Could you check a few things on this model? Use its own coordinates, in mm. A direction names the side the tool comes from. Give positions to 0.01 mm unless a question says otherwise; leave off trailing zeros. Loops run counter-clockwise (first coordinate to the right, second up) from the corner with the lowest first, then second, coordinate; pieces in that order, holes last. Notation, with made-up numbers: (2.5, 84.25) - (54.5, 84.25) arc R35 cw to (54.5, 121.25) - close; hole circle Ø4 at (48, 12). An arc over 180 degrees is marked (long way). Use CSV: the item, a comma, the result in double quotes.
from build123d import *

# Parameters (mm, degrees)
SKETCH1_W                         = 25.4
SKETCH1_H                         = 50.8
SKETCH1_W_2                       = 19.05
SKETCH1_H_2                       = 44.45
EXTRUDE_THIN1_DEPTH               = 501.65
F_3_16_0_1875_DIAMETER_HOLE1_D    = 4.7625
F_3_16_0_195_DIAMETER_HOLE1_D     = 4.953
F_3_16_0_195_DIAMETER_HOLE1_DEPTH = 3.175
F_1_4_0_25_DIAMETER_HOLE1_D       = 6.35
F_1_4_0_25_DIAMETER_HOLE1_DEPTH   = 25.4
F_1_4_0_25_DIAMETER_HOLE1_TIP     = 1.907732465
F_1_4_CLEARANCE_HOLE1_D           = 6.7564
F_1_4_CLEARANCE_HOLE1_DEPTH       = 38.1
F_1_4_CLEARANCE_HOLE1_TIP         = 2.029827343


with BuildPart() as part:
    # Sketch1 → Extrude-Thin1 (new body)
    with BuildSketch(Plane.XY):
        Rectangle(SKETCH1_W, SKETCH1_H)
        Rectangle(SKETCH1_W_2, SKETCH1_H_2, mode=Mode.SUBTRACT)
    extrude(amount=EXTRUDE_THIN1_DEPTH)

    # 3/16 (0.1875) Diameter Hole1 (through all)
    with Locations(Plane(origin=(0, 25.4, 495.3), x_dir=(0, 0, 1), z_dir=(0, 1, 0))):
        with Locations((0, 0), (-488.95, 0), (-463.55, 0), (-438.15, 0), (-25.4, 0), (-50.8, 0)):
            Hole(F_3_16_0_1875_DIAMETER_HOLE1_D / 2)

    # 3/16 (0.195) Diameter Hole1
    with Locations(Plane(origin=(0, -25.4, 0), x_dir=(-1, 0, 0), z_dir=(0, -1, 0))):
        with Locations((-3.175, -85.719336228), (3.175, -111.119336228), (-3.175, -136.519336228), (3.175, -161.919336228), (-3.175, -187.319336228), (3.175, -212.719336228), (-3.175, -238.119336228), (3.175, -263.519336228), (-3.175, -288.919336228), (3.175, -314.319336228), (-3.175, -339.719336228), (3.175, -365.119336228), (3.175, -415.919336228), (-3.175, -390.519336228)):
            Hole(F_3_16_0_195_DIAMETER_HOLE1_D / 2, depth=F_3_16_0_195_DIAMETER_HOLE1_DEPTH)

    # 1/4 (0.25) Diameter Hole1
    with Locations(Plane(origin=(0, 25.4, 0), x_dir=(1, 0, 0), z_dir=(0, 1, 0))):
        with Locations((0, -200.464463093), (0, -422.731), (0, -327.481), (0, -86.154539829)):
            Hole(F_1_4_0_25_DIAMETER_HOLE1_D / 2, depth=F_1_4_0_25_DIAMETER_HOLE1_DEPTH)
            with Locations((0, 0, -(F_1_4_0_25_DIAMETER_HOLE1_DEPTH + F_1_4_0_25_DIAMETER_HOLE1_TIP / 2))):  # 118° drill point
                Cone(0, F_1_4_0_25_DIAMETER_HOLE1_D / 2, F_1_4_0_25_DIAMETER_HOLE1_TIP, mode=Mode.SUBTRACT)

    # 1/4 Clearance Hole1
    with Locations(Plane(origin=(-381, 25.4, 250.825), x_dir=(1, 0, 0), z_dir=(0, 1, 0))):
        with Locations((381, 82.55), (381, 98.425), (381, 114.3), (381, -146.05), (381, -130.175), (381, -114.3), (-381, -146.05), (-381, -130.175), (-381, -114.3), (-381, 82.55), (-381, 98.425), (-381, 114.3)):
            Hole(F_1_4_CLEARANCE_HOLE1_D / 2, depth=F_1_4_CLEARANCE_HOLE1_DEPTH)
            with Locations((0, 0, -(F_1_4_CLEARANCE_HOLE1_DEPTH + F_1_4_CLEARANCE_HOLE1_TIP / 2))):  # 118° drill point
                Cone(0, F_1_4_CLEARANCE_HOLE1_D / 2, F_1_4_CLEARANCE_HOLE1_TIP, mode=Mode.SUBTRACT)


solid = part.part
1) Which directions (+Z, -Z, +X, -X, +Y, -Y) give clear straight access to the entire face, cutting with the end or side of a thin tool? Please do faces 1 (the flat face through (0, -22.225, 247)), 2 (the flat face through (12.7, 0, 247)).
Answer below:
face 1,"+Z, -Z"
face 2,"+Z, -Z, +X, +Y, -Y"
2) Suppose I cut it at A-A (y = -17). Please give me the cut outline in (x, z) (3 decimals), plus the area to 3 significant figures.
Answer below:
outline,"(-12.7, 0) - (-9.525, 0) - (-9.525, 501.65) - (-12.7, 501.65) - close; (9.525, 0) - (12.7, 0) - (12.7, 501.65) - (9.525, 501.65) - close"
area,"3,190 mm2"
3) We'd pull the mould along X, two halves only. Please class faces 3 (the flat face through (0, 25.4, 247)), 4 (the flat face through (-9.525, 0, 247)), 5 (the flat face through (-12.7, 0, 247)): +X half, -X half, draft (parallel to the pull), parting line (faces both ways), or undercut.
Answer below:
face 3,"draft"
face 4,"undercut"
face 5,"-X half"
4) I need wall thicknesses on line 1 along Y through (x, z) = (0.25, 457.5) (3 decimals); line 2 along X through (y, z) = (-9, 42) (3 decimals); line 3 along X through (y, z) = (-23, 469). Which ranges of each line are inside material? Lowest first, please.
Answer below:
line 1,"y = -25.4 to -22.225, 22.225 to 25.4"
line 2,"x = -12.7 to -9.525, 9.525 to 12.7"
line 3,"x = -12.7 to -2.2, 2.2 to 12.7"
5) Suppose I cut it at B-B (z = 347.5). Please give me the cut outline in (x, y) (3 decimals).
Answer below:
outline,"(-12.7, -25.4) - (12.7, -25.4) - (12.7, 25.4) - (-12.7, 25.4) - close; hole (-9.525, -22.225) - (9.525, -22.225) - (9.525, 22.225) - (-9.525, 22.225) - close"
6) I'm going to push a flat-ended pin straight in: P1, Ø10, axis at x = -1, z = 315, coming from the -Y side. Where does the tip first touch, or does it pass through?
Answer below:
P1,"stops at y = -25.4"
